Check sheet for the drawn part. Datum: minimum x, y, z corner. Units: mm. A direction names the side the tool comes from. Coordinates: 2 decimals unless noted, no trailing zeros. Loops run counter-clockwise (first coordinate to the right, second up) from the corner with the lowest first, then second, coordinate; pieces in that order, holes last.
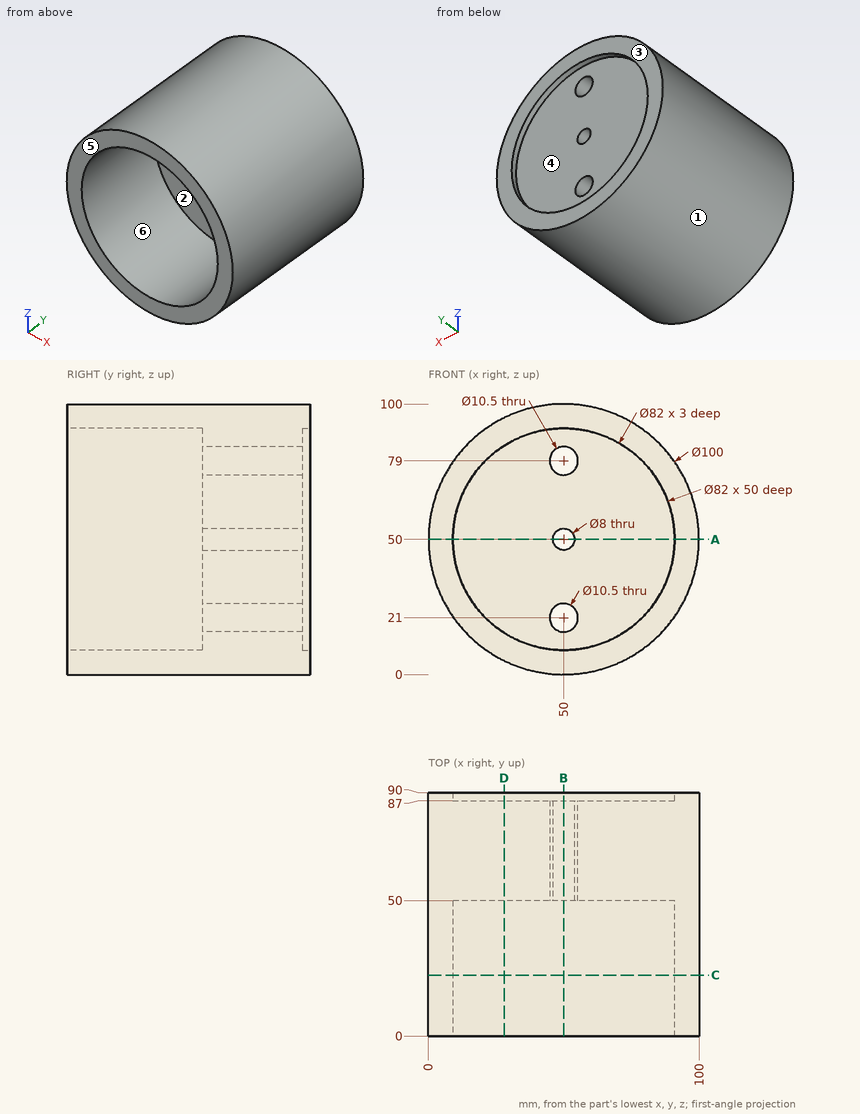
(1) Gauge pin test, flat ends, axial feed: pin 1 Ø4 at (x, y) = (76.5, 39.5) entering from -Z; pin 2 Ø2 at (x, y) = (66, 37) entering from -Z; pin 3 Ø3 at (x, z) = (52, 60.5) entering from -Y. Record the tip position at first contact, or that the pin passes through.
Findings:
pin 1: stops at z = 6.41
pin 2: stops at z = 2.3
pin 3: stops at y = 50
(2) Sectioned sample at D-D on x = 28. Record the cut outline in (y, z).
Findings:
outline: (0, 5.1) - (90, 5.1) - (90, 15.4) - (87, 15.4) - (87, 84.6) - (90, 84.6) - (90, 94.9) - (0, 94.9) - (0, 84.6) - (50, 84.6) - (50, 15.4) - (0, 15.4) - close
(3) Sectioned sample at B-B on x = 50. Record the cut outline in (y, z).
Findings:
outline: (0, 0) - (90, 0) - (90, 9) - (87, 9) - (87, 15.75) - (50, 15.75) - (50, 9) - (0, 9) - close; (0, 91) - (50, 91) - (50, 84.25) - (87, 84.25) - (87, 91) - (90, 91) - (90, 100) - (0, 100) - close; (50, 26.25) - (87, 26.25) - (87, 46) - (50, 46) - close; (50, 54) - (87, 54) - (87, 73.75) - (50, 73.75) - close
(4) Access from +Z, -Z, +X, -X, +Y, -Y to the whole of each face (thin tool, end or side, straight path). Record for the marked faces 4, 5 and 6.
Findings:
face 4: +Y
face 5: +Z, -Z, +X, -X, -Y
face 6: -Y
(5) Draft check along X on the marked faces 1, 2 and 3. Enter one of: +X half, -X half, draft (parallel to the pull), parting line (faces both ways), or undercut.
Findings:
face 1: parting line
face 2: undercut
face 3: draft
(6) Sectioned sample at C-C on y = 22.5. Record the cut outline in (x, z), and give its area (3 significant figures).
Findings:
outline: circle Ø100 at (50, 50); hole circle Ø82 at (50, 50)
area: 2,570 mm2
(7) Scan lines: L1, parallel to Z at x = 50, y = 69.5; L2, parallel to Y at x = 71, z = 69; L3, parallel to X at y = 15, z = 54. Record each from-to range of solid material in increasing order.
Findings:
L1: z = 0 to 15.75, 26.25 to 46, 54 to 73.75, 84.25 to 100
L2: y = 50 to 87
L3: x = 0.16 to 9.2, 90.8 to 99.84
(8) Sectioned sample at A-A on z = 50. Record the cut outline in (x, y), and give its area (3 significant figures).
Findings:
outline: (0, 0) - (9, 0) - (9, 50) - (46, 50) - (46, 87) - (9, 87) - (9, 90) - (0, 90) - close; (54, 50) - (91, 50) - (91, 0) - (100, 0) - (100, 90) - (91, 90) - (91, 87) - (54, 87) - close
area: 4,360 mm2
